Geometry check sheet. Reference: drawing and pictorial views, mm from the part's lowest x, y, z. A direction names the side the tool comes from. Round coordinates to 2 decimals unless told otherwise and drop trailing zeros. Write each loop counter-clockwise with the first axis right and the second up, starting at its lowest first coordinate (ties: lowest second). Pieces come first, ordered by that corner, then holes. Notation, with made-up numbers: M 56.5,84 L 60.5,84 A19 cw 60.5,97 Z; hole C 64,0.25 d1. An arc over 180 degrees is marked long. Use a Markdown table: item, result. Add a question column.
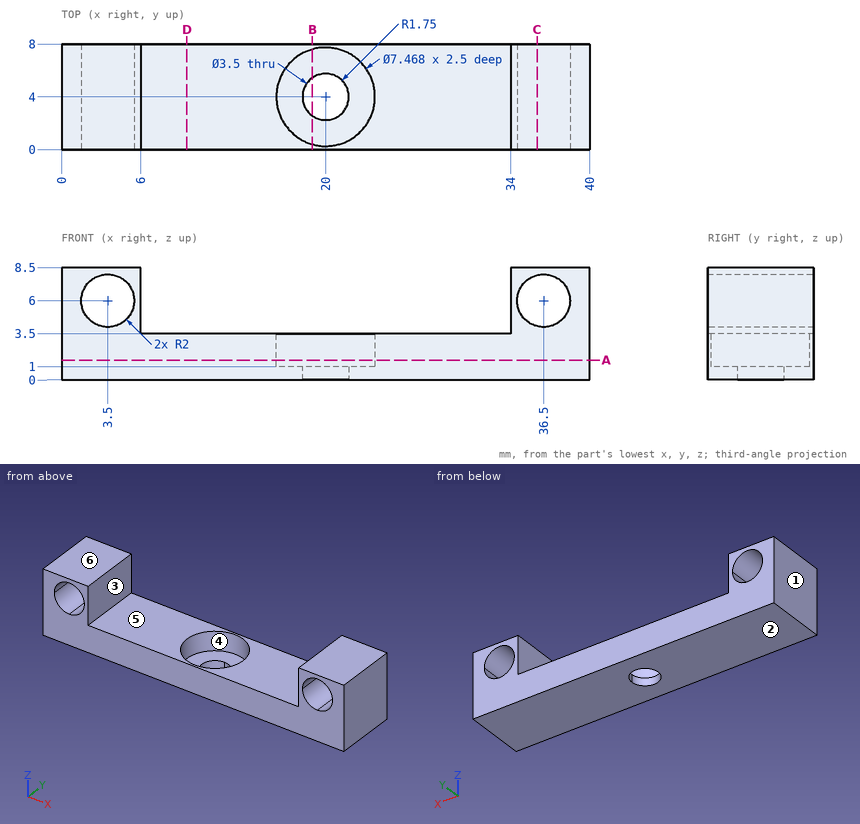
1. Cross-section at C-C on x = 36. Enter the section's corners in (y, z).
2. Scan lines: line 1 along Y through (x, z) = (20, 1.75); line 2 along X through (y, z) = (0.75, 7.75) (1 decimal); line 3 along X through (y, z) = (3.75, 2.5) (1 decimal). Record each from-to range of solid material in increasing order. Write a range as from..to.
3. Access from +Z, -Z, +X, -X, +Y, -Y to the whole of each face (thin tool, end or side, straight path). Record for the marked faces 4, 5 and 6.
4. Release check for a two-part mould opening along X. For the marked faces 1, 2 and 3 record: +X half, -X half, draft (parallel to the pull), parting line (faces both ways), or undercut.
5. Cross-section at A-A on z = 1.5. Enter the section's corners in (x, y).
6. Cross-section at B-B on x = 19. Enter the section's corners in (y, z).
7. Depth check by flat-ended pin: pin 1 Ø2.5 at (x, y) = (26.5, 5) entering from +Z; pin 2 Ø2 at (x, y) = (19.5, 5.5) entering from +Z; pin 3 Ø2 at (x, y) = (20, 4) entering from +Z. Enter the tip coordinate at first touch or a pass-through.
8. Cross-section at D-D on x = 9.5. Enter the section's corners in (y, z), plus the area to 3 significant figures.
Answer:
| question | item | result |
|---|---|---|
| 1 | outline | M 0,0 L 8,0 L 8,4.06 L 0,4.06 Z; M 0,7.94 L 8,7.94 L 8,8.5 L 0,8.5 Z |
| 2 | line 1 | y = 0..0.27, 7.73..8 |
| 2 | line 2 | x = 0..2.5, 4.5..6, 34..35.5, 37.5..40 |
| 2 | line 3 | x = 0..16.3, 23.7..40 |
| 3 | face 4 | +Z |
| 3 | face 5 | +Z, +Y, -Y |
| 3 | face 6 | +Z, +X, -X, +Y, -Y |
| 4 | face 1 | -X half |
| 4 | face 2 | draft |
| 4 | face 3 | undercut |
| 5 | outline | M 0,0 L 40,0 L 40,8 L 0,8 Z; hole C 20,4 d7.47 |
| 6 | outline | M 0,0 L 2.56,0 L 2.56,1 L 0.4,1 L 0.4,3.5 L 0,3.5 Z; M 5.44,0 L 8,0 L 8,3.5 L 7.6,3.5 L 7.6,1 L 5.44,1 Z |
| 7 | pin 1 | stops at z = 3.5 |
| 7 | pin 2 | stops at z = 1 |
| 7 | pin 3 | passes through |
| 8 | outline | M 0,0 L 8,0 L 8,3.5 L 0,3.5 Z |
| 8 | area | 28.0 mm^2 |
